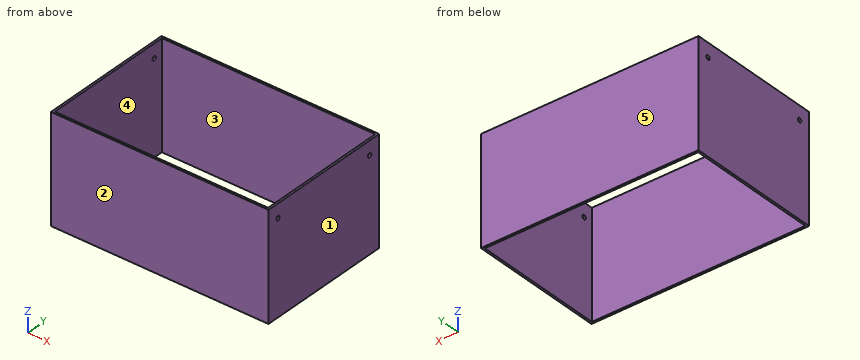
from build123d import *

# Parameters (mm, degrees)
SKETCH_1_W               = 102
SKETCH_1_H               = 64
SKETCH_1_W_2             = 100
SKETCH_1_H_2             = 62
EXTRUDE_1_DEPTH          = 50
CUT_EXTRUDE_2_DEPTH      = 102
CUT_EXTRUDE_2_DEPTH_BACK = 1
SKETCH_5_R               = 1


with BuildPart() as part:
    # Эскиз1 → Бобышка-Вытянуть1 (new body)
    with BuildSketch(Plane.XY):
        with Locations((53, 34)):
            Rectangle(SKETCH_1_W, SKETCH_1_H)
        with Locations((53, 34)):
            Rectangle(SKETCH_1_W_2, SKETCH_1_H_2, mode=Mode.SUBTRACT)
    extrude(amount=EXTRUDE_1_DEPTH)

    # Эскиз5 → Вырез-Вытянуть2 (cut, two sides: drawn at the far end of the back side and taken through both)
    with BuildSketch(Plane.ZY.offset(-103).offset(-CUT_EXTRUDE_2_DEPTH_BACK)):
        with Locations((43.5, 7.5)):
            Circle(SKETCH_5_R)
        with Locations((43.5, 60.5)):
            Circle(SKETCH_5_R)
    extrude(amount=CUT_EXTRUDE_2_DEPTH + CUT_EXTRUDE_2_DEPTH_BACK, mode=Mode.SUBTRACT)


solid = part.part
Could you check a few things on this model? Use its own coordinates, in mm. Face numbers are marked on the shaded views. A direction names the side the tool comes from. Give positions to 0.01 mm unless a question says otherwise; leave off trailing zeros. Order: outer loops, then holes, each group sorted by start corner. A loop starts at its lowest first (then second) coordinate and runs counter-clockwise, first axis right, second up.
Item 1: If we section it at C-C, the plane z = 15: Write out the boundary of the cut face in (x, y).
Item 2: If we mould it in two halves opening along X, with no side actions, what happens to the marked faces 1, 2 and 3? For each: pulls with the +X half, pulls with the -X half, needs draft (parallel to the pull), parting line crosses it, or undercut.
Item 3: If we section it at B-B, the plane y = 32: Write out the boundary of the cut face in (x, z).
Item 4: I'm going to push a flat-ended pin straight in: pin 1 (1.6 mm diameter, centred on y = 7.5, z = 43.5, fed in from -X). Where does the tip first touch, or does it pass through?
Item 5: For the marked faces 4 and 5, which set-ups out of +Z, -Z, +X, -X, +Y, -Y let a thin tool reach every point of the face, with its end or its side?
Item 6: If we section it at A-A, the plane x = 22: Write out the boundary of the cut face in (y, z), plus the area to 3 significant figures.
Item 7: I need wall thicknesses on line 1 (Y direction, x = 103.4, z = 43.5); line 2 (X direction, y = 6, z = 11); line 3 (Y direction, x = 81, z = 15.5). Which ranges of each line are inside material? Lowest first, please.
Values:
1. outline: (2, 2) - (104, 2) - (104, 66) - (2, 66) - close; hole (3, 3) - (103, 3) - (103, 65) - (3, 65) - close
2. face 1: pulls with the +X half
2. face 2: needs draft
2. face 3: undercut
3. outline: (2, 0) - (3, 0) - (3, 50) - (2, 50) - close; (103, 0) - (104, 0) - (104, 50) - (103, 50) - close
4. pin 1: passes through
5. face 4: +Z, -Z
5. face 5: +Z, -Z, +X, -X, +Y
6. outline: (2, 0) - (3, 0) - (3, 50) - (2, 50) - close; (65, 0) - (66, 0) - (66, 50) - (65, 50) - close
6. area: 100 mm2
7. line 1: y = 2 to 6.5, 8.5 to 59.5, 61.5 to 66
7. line 2: x = 2 to 3, 103 to 104
7. line 3: y = 2 to 3, 65 to 66
